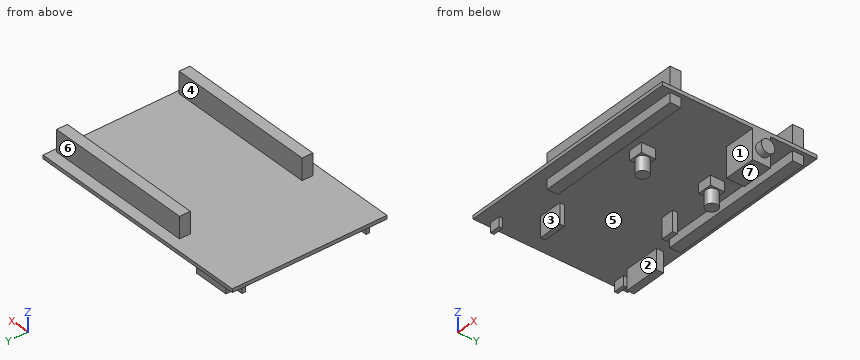
from build123d import *

# Parameters (mm, degrees)
SKETCH1_W                = 97
SKETCH1_H                = 65
BOSS_EXTRUDE1_DEPTH      = 1.5
SKETCH2_W                = 63
SKETCH2_H                = 4.5
BOSS_EXTRUDE2_DEPTH      = 4
BOSS_EXTRUDE2_DEPTH_BACK = 10.5
SKETCH3_W                = 13.5
SKETCH3_H                = 7.5
BOSS_EXTRUDE3_DEPTH      = 12.5
SKETCH4_R                = 2.8
BOSS_EXTRUDE4_DEPTH      = 3
SKETCH5_W                = 4.5
SKETCH5_H                = 1.5
BOSS_EXTRUDE5_DEPTH      = 4
SKETCH6_W                = 15.1
SKETCH6_H                = 3
BOSS_EXTRUDE6_DEPTH      = 8.5
SKETCH7_W                = 10
SKETCH7_H                = 2
BOSS_EXTRUDE7_DEPTH      = 8.5
SKETCH8_W                = 5.5
SKETCH8_H                = 2
BOSS_EXTRUDE8_DEPTH      = 8.5
SKETCH9_W                = 6
SKETCH9_H                = 6
BOSS_EXTRUDE9_DEPTH      = 4
SKETCH10_R               = 2.5
BOSS_EXTRUDE10_DEPTH     = 6
SKETCH13_R               = 2.5
BOSS_EXTRUDE11_DEPTH     = 6


with BuildPart() as part:
    # Sketch1 → Boss-Extrude1 (new body)
    with BuildSketch(Plane.XY):
        Rectangle(SKETCH1_W, SKETCH1_H)
    extrude(amount=BOSS_EXTRUDE1_DEPTH)

    # Sketch2 → Boss-Extrude2 (add, two sides)
    with BuildSketch(Plane(origin=(0, 0, 0), x_dir=(-1, 0, 0), z_dir=(0, 0, -1))) as boss_extrude2_sk:
        with Locations((-15.5, 25.75)):
            Rectangle(SKETCH2_W, SKETCH2_H)
        with Locations((-15.5, -25.75)):
            Rectangle(SKETCH2_W, SKETCH2_H)
    extrude(amount=BOSS_EXTRUDE2_DEPTH)
    extrude(boss_extrude2_sk.sketch, amount=-BOSS_EXTRUDE2_DEPTH_BACK)

    # Sketch3 → Boss-Extrude3 (add)
    with BuildSketch(Plane(origin=(0, 0, 0), x_dir=(-1, 0, 0), z_dir=(0, 0, -1))):
        with Locations((-41.75, 9.25)):
            Rectangle(SKETCH3_W, SKETCH3_H)
    extrude(amount=BOSS_EXTRUDE3_DEPTH)

    # Sketch4 → Boss-Extrude4 (add)
    with BuildSketch(Plane(origin=(48.5, 0, 0), x_dir=(0, 0, -1), z_dir=(1, 0, 0))):
        with Locations((7, 9.5)):
            Circle(SKETCH4_R)
    extrude(amount=BOSS_EXTRUDE4_DEPTH)

    # Sketch5 → Boss-Extrude5 (add)
    with BuildSketch(Plane(origin=(0, 0, 0), x_dir=(-1, 0, 0), z_dir=(0, 0, -1))):
        with Locations((44.25, -26.080181332)):
            Rectangle(SKETCH5_W, SKETCH5_H)
        with Locations((44.25, 26.080181332)):
            Rectangle(SKETCH5_W, SKETCH5_H)
    extrude(amount=BOSS_EXTRUDE5_DEPTH)

    # Sketch6 → Boss-Extrude6 (add)
    with BuildSketch(Plane(origin=(0, 0, 0), x_dir=(-1, 0, 0), z_dir=(0, 0, -1))):
        with Locations((30.95, 25.5)):
            Rectangle(SKETCH6_W, SKETCH6_H)
    extrude(amount=BOSS_EXTRUDE6_DEPTH)

    # Sketch7 → Boss-Extrude7 (add)
    with BuildSketch(Plane(origin=(0, 0, 0), x_dir=(-1, 0, 0), z_dir=(0, 0, -1))):
        with Locations((28.5, -15.5)):
            Rectangle(SKETCH7_W, SKETCH7_H)
    extrude(amount=BOSS_EXTRUDE7_DEPTH)

    # Sketch8 → Boss-Extrude8 (add)
    with BuildSketch(Plane(origin=(0, 0, 0), x_dir=(-1, 0, 0), z_dir=(0, 0, -1))):
        with Locations((6.25, 15.5)):
            Rectangle(SKETCH8_W, SKETCH8_H)
    extrude(amount=BOSS_EXTRUDE8_DEPTH)

    # Sketch9 → Boss-Extrude9 (add)
    with BuildSketch(Plane(origin=(0, 0, 0), x_dir=(-1, 0, 0), z_dir=(0, 0, -1))):
        with Locations((-16.5, -14.5)):
            Rectangle(SKETCH9_W, SKETCH9_H)
        with Locations((-16.5, 14.5)):
            Rectangle(SKETCH9_W, SKETCH9_H)
    extrude(amount=BOSS_EXTRUDE9_DEPTH)

    # Sketch10 → Boss-Extrude10 (add)
    with BuildSketch(Plane(origin=(0, 0, -4), x_dir=(-1, 0, 0), z_dir=(0, 0, -1))):
        with Locations((-16.5, 14.5)):
            Circle(SKETCH10_R)
    extrude(amount=BOSS_EXTRUDE10_DEPTH)

    # Sketch13 → Boss-Extrude11 (add)
    with BuildSketch(Plane(origin=(0, 0, -4), x_dir=(-1, 0, 0), z_dir=(0, 0, -1))):
        with Locations((-16.5, -14.5)):
            Circle(SKETCH13_R)
    extrude(amount=BOSS_EXTRUDE11_DEPTH)


solid = part.part
Read the model definition and answer for the solid it produces. Units are mm, in the model's axes. Face numbers are marked on the shaded views. A direction names the side the tool comes from. Give positions to 0.01 mm unless a question says otherwise; leave off trailing zeros. Loops run counter-clockwise (first coordinate to the right, second up) from the corner with the lowest first, then second, coordinate; pieces in that order, holes last. Notation, with made-up numbers: (48.5, -26.5) - (96.5, -26.5) arc R24 cw to (96.5, 2.5) - close; hole circle Ø4 at (39.5, 67.25). An arc over 180 degrees is marked (long way). Answer as CSV lines item,"result". Start each with the question number.
1) Find section D-D (y = -10). Write down the section's boundary in (x, z), then the cut area to 4 significant figures.
2) Find section A-A (z = 5). Write down the section's boundary in (x, y).
3) Find section C-C (x = -27). Write down the section's boundary in (y, z), then the cut area to 3 significant figures.
4) Which of the six approach directions +Z, -Z, +X, -X, +Y, -Y give full straight-line access (tool end or side, diameter ignored) to the marked faces 1, 2, 3 and 4?
5) Straight lines are drawn through the part: L1, parallel to Y at x = -28, z = -3; L2, parallel to Y at x = 1, z = 7.25; L3, parallel to Z at x = 4, y = -17. For each, find the intervals that lie inside material, in ascending order. Write a range as from..to.
6) Find section B-B (z = -7). Write down the section's boundary in (x, y), then the cut area to 3 significant figures.
7) Each of these flat-tipped pins is pushed along its axis until it touches: pin 1 Ø1.5 at (x, z) = (-13.5, -4.5) entering from -Y; pin 2 Ø4 at (x, y) = (-3.5, 14.5) entering from -Z; pin 3 Ø1.2 at (x, y) = (-45, 26) entering from -Z; pin 4 Ø6 at (x, z) = (-24.5, 7) entering from -Y. Where does it stop, or does it pass through?
8) Determine the mould class of the marked faces 5, 6 and 7 for opening direction Y: released by +Y, released by -Y, zero draft, split by the parting line, or undercut.
Findings below:
1,outline,"(-48.5, 0) - (48.5, 0) - (48.5, 1.5) - (-48.5, 1.5) - close"
1,area,"145.5 mm^2"
2,outline,"(-16, -28) - (47, -28) - (47, -23.5) - (-16, -23.5) - close; (-16, 23.5) - (47, 23.5) - (47, 28) - (-16, 28) - close"
3,outline,"(-32.5, 0) - (-16.5, 0) - (-16.5, -8.5) - (-14.5, -8.5) - (-14.5, 0) - (24, 0) - (24, -8.5) - (27, -8.5) - (27, 0) - (32.5, 0) - (32.5, 1.5) - (-32.5, 1.5) - close"
3,area,"140 mm^2"
4,face 1,"-Z, +X, -X"
4,face 2,"-Z, -X"
4,face 3,"-Z, -X, -Y"
4,face 4,"+Z, +X, -X"
5,L1,"-16.5..-14.5, 24..27"
5,L2,"-28..-23.5, 23.5..28"
5,L3,"0..1.5"
6,outline,"(-38.5, 24) - (-23.4, 24) - (-23.4, 27) - (-38.5, 27) - close; (-33.5, -16.5) - (-23.5, -16.5) - (-23.5, -14.5) - (-33.5, -14.5) - close; (-9, 14.5) - (-3.5, 14.5) - (-3.5, 16.5) - (-9, 16.5) - close; circle Ø5 at (16.5, -14.5); circle Ø5 at (16.5, 14.5); (35, 5.5) - (48.5, 5.5) - (48.5, 6.7) - (51.5, 6.7) - (51.5, 12.3) - (48.5, 12.3) - (48.5, 13) - (35, 13) - close"
6,area,"234 mm^2"
7,pin 1,"y = -28"
7,pin 2,"z = -8.5"
7,pin 3,"z = -4"
7,pin 4,"through"
8,face 5,"undercut"
8,face 6,"released by +Y"
8,face 7,"zero draft"
